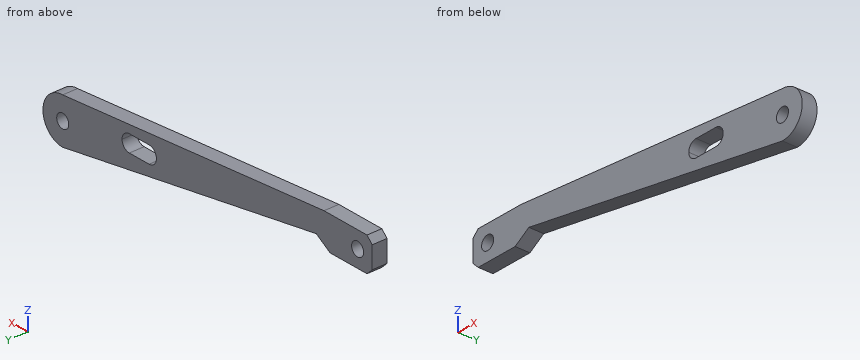
from build123d import *

# Parameters (mm, degrees)
F0_R     = 7
F1_DEPTH = 15


with BuildPart() as f1:
    # F0 (on Front) → F1 (new body)
    with BuildSketch(Plane.XZ):
        with BuildLine():
            Line((285.148505, 27.021557), (-18.851495, 55.021557))
            Line((-18.851495, 55.021557), (-68.851495, 55.021557))
            Line((-68.851495, 55.021557), (-74.851495, 49.021557))
            Line((-74.851495, 49.021557), (-74.851495, 27.021557))
            Line((-74.851495, 27.021557), (-68.851495, 21.021557))
            Line((-68.851495, 21.021557), (-25.851495, 21.021557))
            Line((-25.851495, 21.021557), (-9.851495, 31.021557))
            Line((-9.851495, 31.021557), (285.148505, -18.978443))
            ThreePointArc((285.148505, -18.978443), (308.148505, 4.021557), (285.148505, 27.021557))
        make_face()
        with BuildLine():
            ThreePointArc((176.148505, 17.521557), (178.638097, 23.531965), (184.648505, 26.021557))
            Line((184.648505, 26.021557), (207.648505, 26.021557))
            ThreePointArc((207.648505, 26.021557), (213.658912, 23.531965), (216.148505, 17.521557))
            ThreePointArc((216.148505, 17.521557), (213.658912, 11.51115), (207.648505, 9.021557))
            Line((207.648505, 9.021557), (184.648505, 9.021557))
            ThreePointArc((184.648505, 9.021557), (178.638097, 11.51115), (176.148505, 17.521557))
        make_face(mode=Mode.SUBTRACT)
        with Locations((285.148505, 4.021557)):
            Circle(F0_R, mode=Mode.SUBTRACT)
        with Locations((-57.851495, 38.021557)):
            Circle(F0_R, mode=Mode.SUBTRACT)
    extrude(amount=F1_DEPTH)


solid = f1.part
Model file for the job. Use its own axes, mm. Give positions to 0.01 mm unless a question says otherwise; leave off trailing zeros. Order: outer loops, then holes, each group sorted by start corner. A loop starts at its lowest first (then second) coordinate and runs counter-clockwise, first axis right, second up. Notation, with made-up numbers: (5, -12) - (58, -12) arc R14 cw to (58, -1) - close; hole circle Ø4 at (54, 3.5). An arc over 180 degrees is marked (long way). Return JSON: item names as keys, results as strings.
1) Probe line 1 (Z direction, x = 284.5, y = -3.25); line 2 (Z direction, x = 24.5, y = -3.75); line 3 (Z direction, x = 61.5, y = -6.75). List the from-to ranges inside material, lowest first. Write a range as from..to.
Geometry says:
{"line 1": "-18.87..-2.95, 10.99..27.08", "line 2": "25.2..51.03", "line 3": "18.93..47.62"}
2) Cut at D-D, the plane x = 145.5. Give the cut face in (y, z), plus the area to 3 significant figures.
Geometry says:
{"outline": "(-15, 4.69) - (0, 4.69) - (0, 39.88) - (-15, 39.88) - close", "area": "528 mm²"}
3) Flat gauge pins, fed straight in: P1, Ø4.5, axis at x = -44.5, y = -4, coming from the -Z side; P2, Ø22.5, axis at x = 285.15, z = 4.02, coming from the -Y side; P3, Ø10, axis at x = -24.5, z = 13.5, coming from the +Y side; P4, Ø1.5, axis at x = 135, y = -5.5, coming from the +Z side. Where does each tip first touch, or does it go through?
Geometry says:
{"P1": "z = 21.02", "P2": "y = -15", "P3": "through", "P4": "z = 40.92"}
4) Cut at A-A, the plane y = -7. Give the cut face in (x, z).
Geometry says:
{"outline": "(-74.85, 27.02) - (-68.85, 21.02) - (-25.85, 21.02) - (-9.85, 31.02) - (285.15, -18.98) arc R23 ccw to (285.15, 27.02) - (-18.85, 55.02) - (-68.85, 55.02) - (-74.85, 49.02) - close; hole circle Ø14 at (-57.85, 38.02); hole (176.15, 17.52) arc R8.5 ccw to (184.65, 9.02) - (207.65, 9.02) arc R8.5 ccw to (216.15, 17.52) arc R8.5 ccw to (207.65, 26.02) - (184.65, 26.02) arc R8.5 ccw to start; hole circle Ø14 at (285.15, 4.02)"}
5) Cut at B-B, the plane x = 203. Give the cut face in (y, z).
Geometry says:
{"outline": "(-15, -5.05) - (0, -5.05) - (0, 9.02) - (-15, 9.02) - close; (-15, 26.02) - (0, 26.02) - (0, 34.59) - (-15, 34.59) - close"}
6) Cut at C-C, the plane z = -12. Give the cut face in (x, y).
Geometry says:
{"outline": "(243.98, -15) - (301.65, -15) - (301.65, 0) - (243.98, 0) - close"}
